from build123d import *

# Parameters (mm, degrees)
SKETCH020_W   = 2.93428
SKETCH020_H   = 1
SKETCH021_W   = 2.93428
SKETCH021_H   = 1
SKETCH017_R   = 35
SKETCH017_R_2 = 2.5
SKETCH017_R_3 = 3.5
PAD_DEPTH     = 4
SKETCH018_R   = 20
PAD015_DEPTH  = 4


with BuildPart() as bearing_race_differential:
    # Sketch020 → Revolution008 (revolve)
    with BuildSketch(Plane(origin=(0, 33, -0.5), x_dir=(1, 0, 0), z_dir=(0, -1, 0))):
        with Locations((12.444345, -1)):
            Rectangle(SKETCH020_W, SKETCH020_H)
    revolve(axis=Axis((0, 33, -0.5), (0, 0, 1)))


with BuildPart() as bearing_races:
    # Sketch021 → Revolution009 (revolve)
    with BuildSketch(Plane(origin=(0, 0, -0.5), x_dir=(1, 0, 0), z_dir=(0, -1, 0))):
        with Locations((5.324198, -1)):
            Rectangle(SKETCH021_W, SKETCH021_H)
    revolve(axis=Axis((0, 0, -0.5), (0, 0, 1)))

    # Fusion015: union bearing race - differential
    add(bearing_race_differential.part)


with BuildPart() as main:
    # Sketch017 → Pad (new body)
    with BuildSketch(Plane.XY.offset(-1)):
        Circle(SKETCH017_R)
        with Locations((24, 0)):
            Circle(SKETCH017_R_2, mode=Mode.SUBTRACT)
        Circle(SKETCH017_R_3, mode=Mode.SUBTRACT)
        with BuildLine():
            ThreePointArc((-26.499998, 0.011018), (-18.746119, -18.730537), (-0.011018, -26.499998))
            ThreePointArc((-0.011018, -26.499998), (2.490021, -24.001037), (-0.008939, -21.499998))
            ThreePointArc((-21.499998, 0.008939), (-15.209115, -15.196474), (-0.008939, -21.499998))
            ThreePointArc((-21.499998, 0.008939), (-23.998959, 2.509978), (-26.499998, 0.011018))
        make_face(mode=Mode.SUBTRACT)
    extrude(amount=-PAD_DEPTH)


with BuildPart() as cut011002005:
    # Sketch018 → Pad015 (new body)
    with BuildSketch(Plane.XY.offset(-1)):
        with Locations((0, 33)):
            Circle(SKETCH018_R)
    extrude(amount=-PAD015_DEPTH)

    # Fusion: union Main
    add(main.part)

    # Cut011002005: cut bearing races
    add(bearing_races.part, mode=Mode.SUBTRACT)


solid = cut011002005.part
For this review, take the finished solid that the model builds, in its own axes (mm). A direction names the side the tool comes from. Give positions to 0.01 mm unless a question says otherwise; leave off trailing zeros. Order: outer loops, then holes, each group sorted by start corner. A loop starts at its lowest first (then second) coordinate and runs counter-clockwise, first axis right, second up. Notation, with made-up numbers: M -39.5,-13 L -35.5,-13 A19 ccw -35.5,22 Z; hole C 70.25,17 d6. An arc over 180 degrees is marked long. Answer in a Markdown table with one row per item. Add a question column.
(1) Consider section C-C on z = -2.85. State the section outline as (x, y) points.
(2) For pin 1 (6 mm diameter, centred on x = 24, y = 0, fed in from +Z); pin 2 (1.5 mm diameter, centred on y = 40, z = -1.5, fed in from +X), all flat-tipped, find the tip position at first contact; note any pin that passes through.
(3) Mouldability with a two-part tool opening along X and no side actions: class faces 1 (the face through (-3.02, 19.42, -1.49)), 2 (the face through (0, 10, -1)), 3 (the face through (0, 53, -3)) as +X half, -X half, draft (parallel to the pull), parting line (faces both ways), or undercut.
(4) Consider section D-D on y = 33. State the section outline as (x, z) points, and give its area (3 significant figures).
(5) Consider section B-B on x = 24. State the section outline as (y, z) points, and give its area (3 significant figures).
(6) Wall thickness on probe 1 along Y at (x, z) = (0, -3.15); probe 2 along Y at (x, z) = (-17.5, -2.85); probe 3 along Y at (x, z) = (24, -2.25): over which ranges is each line inside the solid? List them lowest first. Write a range as [from, to].
(7) Consider section A-A on y = -24.5. State the section outline as (x, z) points (1 decimal).
(8) For faces 4 (the face through (2.49, -24.06, -2.97)), 5 (the face through (0, 33, -1)), 6 (the face through (10.4, 28.9, -2)), list the 3-axis set-ups (+Z, -Z, +X, -X, +Y, -Y) from which the entire face can be reached by the end or side of a thin tool; tool diameter is ignored.
Evaluation:
| question | item | result |
|---|---|---|
| 1 | outline | M -19.6,29 A35 ccw long 19.6,29 A20 ccw long Z; hole M -26.5,0.01 A26.5 ccw -0.01,-26.5 A2.5 ccw -0.01,-21.5 A21.5 cw -21.5,0.01 A2.5 ccw Z; hole C 0,0 d7; hole C 24,0 d5 |
| 2 | pin 1 | stops at z = -1 |
| 2 | pin 2 | stops at x = 19 |
| 3 | face 1 | undercut |
| 3 | face 2 | draft |
| 3 | face 3 | parting line |
| 4 | outline | M -20,-5 L 20,-5 L 20,-1 L 13.91,-1 L 13.91,-2 L 10.98,-2 L 10.98,-1 L -10.98,-1 L -10.98,-2 L -13.91,-2 L -13.91,-1 L -20,-1 Z |
| 4 | area | 154 mm^2 |
| 5 | outline | M -25.48,-5 L -2.5,-5 L -2.5,-1 L -25.48,-1 Z; M 2.5,-5 L 25.48,-5 L 25.48,-1 L 2.5,-1 Z |
| 5 | area | 184 mm^2 |
| 6 | probe 1 | y = [-35, -26.5], [-21.5, -3.5], [3.5, 53] |
| 6 | probe 2 | y = [-30.31, -19.9], [-12.49, 42.68] |
| 6 | probe 3 | y = [-25.48, -2.5], [2.5, 25.48] |
| 7 | outline | M -25,-5 L -10.1,-5 L -10.1,-1 L -25,-1 Z; M 2.4,-5 L 25,-5 L 25,-1 L 2.4,-1 Z |
| 8 | face 4 | +Z, -Z |
| 8 | face 5 | +Z, +X, -X, +Y, -Y |
| 8 | face 6 | +Z |
